```python
from build123d import *

# Parameters (mm, degrees)
SZKIC1_R                    = 3.000000079
DODANIE_WYCI_GNI_CIE1_DEPTH = 5
SZKIC2_W                    = 105.552332286
SZKIC2_H                    = 7.505645785
SZKIC2_W_2                  = 0.651830256
SZKIC2_H_2                  = 5.051684483
WYTNIJ_WYCI_GNI_CIE3_DEPTH  = 6


with BuildPart() as part:
    # Szkic1 → Dodanie-wyciągnięcie1 (new body)
    with BuildSketch(Plane.XY):
        with BuildLine():
            ThreePointArc((82.288446866, -5.322288535), (88.646994763, 2.576863373), (78.537310202, 1.78818708))
            ThreePointArc((78.537310202, 1.78818708), (77.588574134, 0.574418105), (76.092138721, 0.208335732))
            ThreePointArc((76.092138721, 0.208335732), (41.955082096, 1.834260744), (7.813610577, 0.303839332))
            ThreePointArc((7.813610577, 0.303839332), (5.63200922, 0.736314196), (4.033915145, 2.283089654))
            ThreePointArc((4.033915145, 2.283089654), (-4.263785422, 1.817994402), (1.14538756, -4.491442653))
            ThreePointArc((1.14538756, -4.491442653), (41.771214226, 0.395953927), (82.288446866, -5.322288535))
        make_face()
        Circle(SZKIC1_R, mode=Mode.SUBTRACT)
        with Locations((83.76241555, 0)):
            Circle(SZKIC1_R, mode=Mode.SUBTRACT)
    extrude(amount=DODANIE_WYCI_GNI_CIE1_DEPTH)

    # Szkic2 → Wytnij-wyciągnięcie3 (cut, through all)
    with BuildSketch(Plane.XY):
        with Locations((141.671704443, 0.381285041)):
            Rectangle(SZKIC2_W, SZKIC2_H)
        with Locations((-4.682734605, -0.038745932)):
            Rectangle(SZKIC2_W_2, SZKIC2_H_2)
    extrude(amount=WYTNIJ_WYCI_GNI_CIE3_DEPTH, mode=Mode.SUBTRACT)


solid = part.part
```
Verification items for the finished model (mm, model axes). Coordinates: 2 decimals unless noted, no trailing zeros. Order: outer loops, then holes, each group sorted by start corner. A loop starts at its lowest first (then second) coordinate and runs counter-clockwise, first axis right, second up. Notation, with made-up numbers: (80, 0) -> (116, 0) arc R17 cw to (116, 21) -> close; hole circle Ø2 at (-14, -17). An arc over 180 degrees is marked (long way). Put each result on its own line as item: value. Start each with the question number.
1) Material ranges on L1, parallel to Y at x = 0, z = 2.05; L2, parallel to X at y = 2.5, z = 0.8; L3, parallel to X at y = 4, z = 1.4, recorded low to high.
2) Cross-section at A-A (x = 0). Enter the section's corners in (y, z).
3) Release check for a two-part mould opening along Y. For faces 1 (the cylindrical face through (77.61, 0.59, 2.46)), 2 (the cylindrical face through (41.2, 0.4, 2.5)), 3 (the cylindrical face through (0, 3, 2)) record: pulls with the +Y half, pulls with the -Y half, needs draft (parallel to the pull), parting line crosses it, or undercut.
4) Cross-section at B-B (z = 1.55). Enter the section's corners in (x, y).
5) Cross-section at D-D (x = 41). Enter the section's corners in (y, z).
6) Go/stop test with flat-tipped pins: pin 1 (2 mm diameter, centred on x = 53.5, z = 1.5, fed in from -Y); pin 2 (3.5 mm diameter, centred on x = 83.76, y = 0, fed in from +Z); pin 3 (1.5 mm diameter, centred on x = 61, z = 3.5, fed in from -Y). Record where each tip stops, or that it passes through.
7) Cross-section at C-C (x = 15.5). Enter the section's corners in (y, z).
Geometry check:
1. L1: y = -4.64 to -3, 3 to 4.64
1. L2: x = -3.9 to -1.66, 1.66 to 3.9, 78.84 to 82.1, 85.42 to 88.69
1. L3: x = -2.34 to 2.34, 79.95 to 87.57
2. outline: (-4.64, 0) -> (-3, 0) -> (-3, 5) -> (-4.64, 5) -> close; (3, 0) -> (4.64, 0) -> (4.64, 5) -> (3, 5) -> close
3. face 1: pulls with the +Y half
3. face 2: pulls with the -Y half
3. face 3: undercut
4. outline: (-4.36, -1.58) arc R4.64 ccw to (1.15, -4.49) arc R157.86 cw to (82.29, -5.32) arc R5.52 ccw to (88.9, -2.04) -> (88.9, 2.04) arc R5.52 ccw to (78.54, 1.79) arc R2.35 cw to (76.09, 0.21) arc R370.04 ccw to (7.81, 0.3) arc R3.93 cw to (4.03, 2.28) arc R4.64 ccw to (-4.36, 1.58) -> close; hole circle Ø6 at (0, 0); hole circle Ø6 at (83.76, 0)
5. outline: (0.4, 0) -> (1.83, 0) -> (1.83, 5) -> (0.4, 5) -> close
6. pin 1: stops at y = -0.25
6. pin 2: passes through
6. pin 3: stops at y = -1.08
7. outline: (-1.53, 0) -> (0.92, 0) -> (0.92, 5) -> (-1.53, 5) -> close
